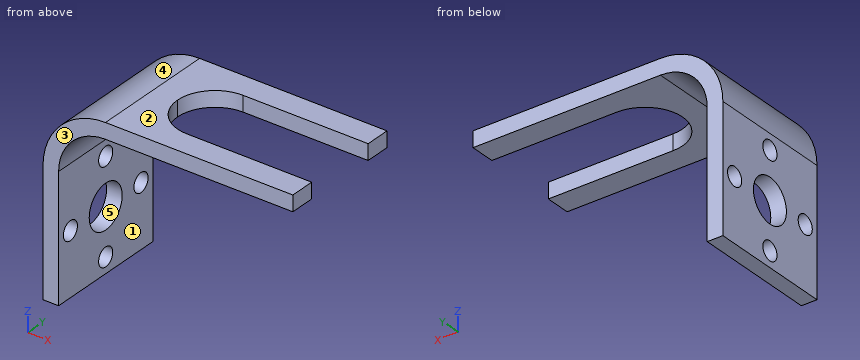
from build123d import *

# Parameters (mm, degrees)
F1_DEPTH = 25.4
F3_DEPTH = 3.175
F4_R     = 4.445
F4_R_2   = 1.905
F5_DEPTH = 3.175


with BuildPart() as f1:
    # F0 (on Front) → F1 (new body)
    with BuildSketch(Plane.XZ):
        with BuildLine():
            Line((0, 25.4), (0, 0))
            Line((0, 0), (3.175, 0))
            Line((3.175, 0), (3.175, 25.4))
            ThreePointArc((3.175, 25.4), (5.964808, 32.135192), (12.7, 34.925))
            Line((12.7, 34.925), (50.8, 34.925))
            Line((50.8, 34.925), (50.8, 38.1))
            Line((50.8, 38.1), (12.7, 38.1))
            ThreePointArc((12.7, 38.1), (3.719744, 34.380256), (0, 25.4))
        make_face()
    extrude(amount=F1_DEPTH)

    # F2 (on face) → F3 (cut, through all)
    with BuildSketch(Plane(origin=(0, 0, 34.925), x_dir=(1, 0, 0), z_dir=(0, 0, -1))):
        with BuildLine():
            Line((50.8, 5.08), (50.8, 20.32))
            Line((50.8, 20.32), (25.4, 20.32))
            ThreePointArc((25.4, 20.32), (20.011846, 18.088154), (17.78, 12.7))
            ThreePointArc((17.78, 12.7), (20.011846, 7.311846), (25.4, 5.08))
            Line((25.4, 5.08), (50.8, 5.08))
        make_face()
    extrude(amount=-F3_DEPTH, mode=Mode.SUBTRACT)

    # F4 (on face) → F5 (cut, through all)
    with BuildSketch(Plane(origin=(0, 0, 0), x_dir=(0, -1, 0), z_dir=(-1, 0, 0))):
        with Locations((12.7, 12.7)):
            Circle(F4_R)
        with Locations((22.225, 12.7)):
            Circle(F4_R_2)
        with Locations((12.7, 3.175)):
            Circle(F4_R_2)
        with Locations((3.175, 12.7)):
            Circle(F4_R_2)
        with Locations((12.7, 22.225)):
            Circle(F4_R_2)
    extrude(amount=-F5_DEPTH, mode=Mode.SUBTRACT)


solid = f1.part
The model under review builds one solid part; all positions refer to its coordinate system, in mm. Face numbers are marked on the shaded views. A direction names the side the tool comes from. Round coordinates to 2 decimals unless told otherwise and drop trailing zeros. Loops run counter-clockwise (first coordinate to the right, second up) from the corner with the lowest first, then second, coordinate; pieces in that order, holes last. Notation, with made-up numbers: (-2.75, -11.5) - (8.25, -11.5) arc R26 ccw to (8.25, 14.5) - close; hole circle Ø5 at (31.25, 1.5). An arc over 180 degrees is marked (long way). Use CSV: the item, a comma, the result in double quotes.
(1) Take a section at D-D, the plane z = 35.5. Give the boundary of the cut face in (x, y), plus the area to 3 significant figures.
Working result:
outline,"(5, -25.4) - (50.8, -25.4) - (50.8, -20.32) - (25.4, -20.32) arc R7.62 cw to (17.78, -12.7) arc R7.62 cw to (25.4, -5.08) - (50.8, -5.08) - (50.8, 0) - (5, 0) - close"
area,"685 mm^2"
(2) The part is to be moulded in two halves that separate along Z. For the marked faces 3, 4 and 5, say which applies: pulls with the +Z half, pulls with the -Z half, needs draft (parallel to the pull), parting line crosses it, or undercut.
Working result:
face 3,"needs draft"
face 4,"pulls with the +Z half"
face 5,"undercut"
(3) For line 1 (Z direction, x = 2.15, y = -12.7) (3 decimals); line 2 (X direction, y = -6.5, z = 18) (3 decimals); line 3 (Z direction, x = 38, y = -23.25) (3 decimals), list the stretches that pass through material, from the lowest coordinate up.
Working result:
line 1,"z = 0 to 1.27, 5.08 to 8.255, 17.145 to 20.32, 24.13 to 32.47"
line 2,"x = 0 to 3.175"
line 3,"z = 34.925 to 38.1"
(4) Machinability: for the marked faces 1 and 2, which of the approach directions +Z, -Z, +X, -X, +Y, -Y give a long, thin tool a straight path to every point of the face, cutting with its end or side? Answer none if there is none.
Working result:
face 1,"-Z, +X, +Y, -Y"
face 2,"+Z, +X, -X, +Y, -Y"
(5) Take a section at B-B, the plane x = 34. Give the boundary of the cut face in (y, z) (3 decimals).
Working result:
outline,"(-25.4, 34.925) - (-20.32, 34.925) - (-20.32, 38.1) - (-25.4, 38.1) - close; (-5.08, 34.925) - (0, 34.925) - (0, 38.1) - (-5.08, 38.1) - close"
(6) Take a section at C-C, the plane x = 18.5. Give the boundary of the cut face in (y, z) (3 decimals).
Working result:
outline,"(-25.4, 34.925) - (-15.933, 34.925) - (-15.933, 38.1) - (-25.4, 38.1) - close; (-9.467, 34.925) - (0, 34.925) - (0, 38.1) - (-9.467, 38.1) - close"
(7) Take a section at A-A, the plane z = 12.7. Give the boundary of the cut face in (x, y) (3 decimals).
Working result:
outline,"(0, -25.4) - (3.175, -25.4) - (3.175, -24.13) - (0, -24.13) - close; (0, -20.32) - (3.175, -20.32) - (3.175, -17.145) - (0, -17.145) - close; (0, -8.255) - (3.175, -8.255) - (3.175, -5.08) - (0, -5.08) - close; (0, -1.27) - (3.175, -1.27) - (3.175, 0) - (0, 0) - close"
(8) Clearance check with flat-ended pins moving along their axes: P1, Ø3.5, axis at x = 33, z = 37, coming from the +Y side; P2, Ø10, axis at y = -17.5, z = 9, coming from the +X side (3 decimals). State where each tip first meets the part, or that it passes through.
Working result:
P1,"stops at y = 0"
P2,"stops at x = 3.175"
